Source: CAD feature listing. Evaluate the final solid. Frame: model axes, mm. Round coordinates to 2 decimals unless told otherwise and drop trailing zeros. Loops run counter-clockwise (first coordinate to the right, second up) from the corner with the lowest first, then second, coordinate; pieces in that order, holes last.
(1) Section C-C, the plane z = 3.5. Return the cut outline in (x, y), plus the area to 3 significant figures.
(2) Material intervals for probe 1 along Y at (x, z) = (0, 3.5); probe 2 along Y at (x, z) = (-8, 3.35); probe 3 along X at (y, z) = (-3, 1.55), sorted ascending.
(3) Section A-A, the plane y = -8. Return the cut outline in (x, z).
(4) Section D-D, the plane x = 0. Return the cut outline in (y, z), plus the area to 3 significant figures.
(5) Mould query, pull axis Y, two halves, no side actions, for faces 1 (the flat face through (15, 45, 2)), 2 (the cylindrical face through (-0.39, -9.757, 2.535)), 3 (the flat face through (-15, 15, 2)), 4 (the cylindrical face through (-9.8, 0.08, 2.54)). Classes: pulls with the +Y half, pulls with the -Y half, needs draft (parallel to the pull), parting line crosses it, or undercut.
```python
from build123d import *

# Parameters (mm, degrees)
SKETCH_W      = 60
SKETCH_H      = 60
PAD_DEPTH     = 5
SKETCH001_R   = 1.8
SKETCH001_R_2 = 5.4
POCKET_DEPTH  = 15


with BuildPart() as part:
    # Sketch → Pad (new body)
    with BuildSketch(Plane.XY):
        with Locations((15, 15)):
            Rectangle(SKETCH_W, SKETCH_H)
    extrude(amount=PAD_DEPTH)

    # Sketch001 (on Face6 of Pad) → Pocket (cut)
    with BuildSketch(Plane.XY.offset(5)):
        with Locations((-8, 0)):
            Circle(SKETCH001_R)
        with Locations((0, -8)):
            Circle(SKETCH001_R)
        with Locations((0, 8)):
            Circle(SKETCH001_R)
        with Locations((8, 0)):
            Circle(SKETCH001_R)
        Circle(SKETCH001_R_2)
        with Locations((30, 0)):
            Circle(SKETCH001_R_2)
    extrude(amount=-POCKET_DEPTH, mode=Mode.SUBTRACT)


solid = part.part
```
Output values:
1. outline: (-15, -15) - (45, -15) - (45, 45) - (-15, 45) - close; hole circle Ø3.6 at (-8, 0); hole circle Ø10.8 at (0, 0); hole circle Ø3.6 at (0, -8); hole circle Ø3.6 at (0, 8); hole circle Ø3.6 at (8, 0); hole circle Ø10.8 at (30, 0)
1. area: 3,380 mm2
2. probe 1: y = -15 to -9.8, -6.2 to -5.4, 5.4 to 6.2, 9.8 to 45
2. probe 2: y = -15 to -1.8, 1.8 to 45
2. probe 3: x = -15 to -4.49, 4.49 to 25.51, 34.49 to 45
3. outline: (-15, 0) - (-1.8, 0) - (-1.8, 5) - (-15, 5) - close; (1.8, 0) - (45, 0) - (45, 5) - (1.8, 5) - close
4. outline: (-15, 0) - (-9.8, 0) - (-9.8, 5) - (-15, 5) - close; (-6.2, 0) - (-5.4, 0) - (-5.4, 5) - (-6.2, 5) - close; (5.4, 0) - (6.2, 0) - (6.2, 5) - (5.4, 5) - close; (9.8, 0) - (45, 0) - (45, 5) - (9.8, 5) - close
4. area: 210 mm2
5. face 1: pulls with the +Y half
5. face 2: undercut
5. face 3: needs draft
5. face 4: undercut
